The listing builds one solid part. Answer for the finished solid, in the listing's coordinates (mm). A direction names the side the tool comes from. Round coordinates to 2 decimals unless told otherwise and drop trailing zeros. Order: outer loops, then holes, each group sorted by start corner. A loop starts at its lowest first (then second) coordinate and runs counter-clockwise, first axis right, second up. Notation, with made-up numbers: (57, 62.25) -> (110, 62.25) arc R14 cw to (110, 84.25) -> close; hole circle Ø4 at (-21, -34.75). An arc over 180 degrees is marked (long way). Answer in a Markdown table with one row per item. Add a question column.
```python
from build123d import *

# Parameters (mm, degrees)
SKETCH1_R              = 10.25
SKETCH1_R_2            = 2
SKETCH1_R_3            = 1.2
BOSS_EXTRUDE1_DEPTH    = 3.5
CUT_EXTRUDE2_START     = -1.7
CUT_EXTRUDE2_OUTLINE_R = 1.2
CUT_EXTRUDE2_DEPTH     = 1.7
SKETCH6_R              = 8
CUT_EXTRUDE4_DEPTH     = 1.7


# Read off the part's stored shape, not the designer's step: Cut-Extrude2
with BuildPart() as part:
    # Sketch1 → Boss-Extrude1 (new body)
    with BuildSketch(Plane.XY):
        Circle(SKETCH1_R)
        Circle(SKETCH1_R_2, mode=Mode.SUBTRACT)
        with Locations((0, 8)):
            Circle(SKETCH1_R_3, mode=Mode.SUBTRACT)
        with Locations((8, 0)):
            Circle(SKETCH1_R_3, mode=Mode.SUBTRACT)
        with Locations((0, -8)):
            Circle(SKETCH1_R_3, mode=Mode.SUBTRACT)
        with Locations((-8, 0)):
            Circle(SKETCH1_R_3, mode=Mode.SUBTRACT)
    extrude(amount=BOSS_EXTRUDE1_DEPTH)

    # Cut-Extrude2 outline → Cut-Extrude2 (cut)
    # profile 1 of 4: a face of its own
    with BuildSketch(Plane(origin=(0, 0, 0), x_dir=(-1, 0, 0), z_dir=(0, 0, -1)).offset(CUT_EXTRUDE2_START)):
        with BuildLine():
            Line((-9.94069912, -2.499), (-8.098979998, -2.499))
            ThreePointArc((-8.098979998, -2.499), (-5.49948025, -0.050000196), (-8.000999999, 2.4989992))
            Line((-8.000999999, 2.4989992), (-9.940699321, 2.4989992))
            ThreePointArc((-9.940699321, 2.4989992), (-10.25, -4.12e-07), (-9.94069912, -2.499))
        make_face()
        with Locations((-8, 0)):
            Circle(CUT_EXTRUDE2_OUTLINE_R, mode=Mode.SUBTRACT)
    # profile 2 of 4: a face of its own
    with BuildSketch(Plane(origin=(0, 0, 0), x_dir=(-1, 0, 0), z_dir=(0, 0, -1)).offset(CUT_EXTRUDE2_START)):
        with BuildLine():
            Line((-2.498, -8), (-2.498, -9.940950458))
            ThreePointArc((-2.498, -9.940950458), (0.001546691, -10.249999883), (2.501, -9.940196125))
            Line((2.501, -9.940196125), (2.5010004, -8.070689462))
            ThreePointArc((2.5010004, -8.070689462), (0.037348265, -5.500249912), (-2.498, -8))
        make_face()
        with Locations((0, -8)):
            Circle(CUT_EXTRUDE2_OUTLINE_R, mode=Mode.SUBTRACT)
    # profile 3 of 4: a face of its own
    with BuildSketch(Plane(origin=(0, 0, 0), x_dir=(-1, 0, 0), z_dir=(0, 0, -1)).offset(CUT_EXTRUDE2_START)):
        with BuildLine():
            ThreePointArc((2.5, 9.940447676), (0, 10.25), (-2.5, 9.940447676))
            Line((-2.5, 9.940447676), (-2.5, 8))
            ThreePointArc((-2.5, 8), (0, 5.5), (2.5, 8))
            Line((2.5, 8), (2.5, 9.940447676))
        make_face()
        with Locations((0, 8)):
            Circle(CUT_EXTRUDE2_OUTLINE_R, mode=Mode.SUBTRACT)
    # profile 4 of 4: a face of its own
    with BuildSketch(Plane(origin=(0, 0, 0), x_dir=(-1, 0, 0), z_dir=(0, 0, -1)).offset(CUT_EXTRUDE2_START)):
        with BuildLine():
            Line((8.001, -2.499), (9.94069912, -2.499))
            ThreePointArc((9.94069912, -2.499), (10.249999948, 0.001031141), (9.940196125, 2.501))
            Line((9.940196125, 2.501), (8.001, 2.501))
            ThreePointArc((8.001, 2.501), (5.501, 0.001), (8.001, -2.499))
        make_face()
        with Locations((8, 0)):
            Circle(CUT_EXTRUDE2_OUTLINE_R, mode=Mode.SUBTRACT)
    extrude(amount=CUT_EXTRUDE2_DEPTH, mode=Mode.SUBTRACT)

    # Sketch6 → Cut-Extrude4 (cut)
    with BuildSketch(Plane(origin=(0, 0, 0), x_dir=(-1, 0, 0), z_dir=(0, 0, -1))):
        Circle(SKETCH6_R)
    extrude(amount=-CUT_EXTRUDE4_DEPTH, mode=Mode.SUBTRACT)


solid = part.part
```
1. Each of these flat-tipped pins is pushed along its axis until it touches: pin 1 (0.8 mm diameter, centred on y = 9, z = 0.5, fed in from +X); pin 2 (0.8 mm diameter, centred on y = 8.5, z = 1, fed in from -X); pin 3 (3 mm diameter, centred on x = 0, y = -8, fed in from -Z). Where does it stop, or does it pass through?
2. Straight lines are drawn through the part: line 1 along Y through (x, z) = (0, 3); line 2 along Z through (x, y) = (7.5, -1.75); line 3 along X through (y, z) = (1.5, 1.75). For each, find the intervals that lie inside material, in ascending order.
3. The part is cut by section D-D (z = 2.4). Give the vertices of the cut face in (x, y), then the cut area to 3 significant figures.
4. The part is cut by section A-A (z = 0.6). Give the vertices of the cut face in (x, y).
5. The mould has two halves that part along Y. Classify faces 1 (the cylindrical face through (9.468, -3.926, 1.726)), 2 (the flat face through (6, -6, 0)), 3 (the cylindrical face through (5.693, -5.621, 0.838)): released by +Y, released by -Y, zero draft, split by the parting line, or undercut.
6. The part is cut by section B-B (x = 0). Give the vertices of the cut face in (y, z).
7. For faces 4 (the cylindrical face through (-5.694, 5.62, 0.838)), 5 (the flat face through (-2.501, -9, 1)), 6 (the flat face through (9, -2.499, 1)), 7 (the flat face through (-9, -2.499, 1)), 8 (the flat face through (-2.5, 9, 1)), determine the directions among +Z, -Z, +X, -X, +Y, -Y from which every point of the face is accessible in a straight line to the end or side of a thin tool.
Report:
| question | item | result |
|---|---|---|
| 1 | pin 1 | stops at x = 5.58 |
| 1 | pin 2 | stops at x = -6.28 |
| 1 | pin 3 | stops at z = 1.7 |
| 2 | line 1 | y = -10.25 to -9.2, -6.8 to -2, 2 to 6.8, 9.2 to 10.25 |
| 2 | line 2 | z = 1.7 to 3.5 |
| 2 | line 3 | x = -10.14 to -1.32, 1.32 to 10.14 |
| 3 | outline | circle Ø20.5 at (0, 0); hole circle Ø2.4 at (-8, 0); hole circle Ø4 at (0, 0); hole circle Ø2.4 at (0, -8); hole circle Ø2.4 at (0, 8); hole circle Ø2.4 at (8, 0) |
| 3 | area | 299 mm^2 |
| 4 | outline | (-9.94, -2.5) arc R10.25 ccw to (-2.5, -9.94) -> (-2.5, -8.07) arc R2.5 cw to (-2.47, -7.61) arc R8 cw to (-7.61, -2.47) arc R2.5 cw to (-8, -2.5) -> close; (-9.94, 2.5) -> (-8, 2.5) arc R2.5 cw to (-7.61, 2.47) arc R8 cw to (-2.47, 7.61) arc R2.5 cw to (-2.5, 8) -> (-2.5, 9.94) arc R10.25 ccw to start; (2.47, -7.61) arc R2.5 cw to (2.5, -8) -> (2.5, -9.94) arc R10.25 ccw to (9.94, -2.5) -> (8.1, -2.5) arc R2.5 cw to (7.61, -2.47) arc R8 cw to start; (2.47, 7.61) arc R8 cw to (7.61, 2.47) arc R2.5 cw to (8, 2.5) -> (9.94, 2.5) arc R10.25 ccw to (2.5, 9.94) -> (2.5, 8) arc R2.5 cw to start |
| 5 | face 1 | split by the parting line |
| 5 | face 2 | zero draft |
| 5 | face 3 | undercut |
| 6 | outline | (-10.25, 1.7) -> (-9.2, 1.7) -> (-9.2, 3.5) -> (-10.25, 3.5) -> close; (-6.8, 1.7) -> (-2, 1.7) -> (-2, 3.5) -> (-6.8, 3.5) -> close; (2, 1.7) -> (6.8, 1.7) -> (6.8, 3.5) -> (2, 3.5) -> close; (9.2, 1.7) -> (10.25, 1.7) -> (10.25, 3.5) -> (9.2, 3.5) -> close |
| 7 | face 4 | -Z |
| 7 | face 5 | -Z, -Y |
| 7 | face 6 | -Z, +X |
| 7 | face 7 | -Z, -X |
| 7 | face 8 | -Z, +Y |
